The model under review builds one solid part; all positions refer to its coordinate system, in mm. Coordinates: 2 decimals unless noted, no trailing zeros. Answer in a Markdown table with one row per item.
```python
from build123d import *

# Parameters (mm, degrees)
SKETCH1_W           = 359.156
SKETCH1_H           = 127
BOSS_EXTRUDE1_DEPTH = 19.05
CUT_EXTRUDE1_REACH  = 21.05
SKETCH2_R           = 2.85115
CUT_EXTRUDE2_REACH  = 21.05
SKETCH3_R           = 3.175


with BuildPart() as part:
    # Sketch1 → Boss-Extrude1 (new body)
    with BuildSketch(Plane.XY):
        with Locations((179.578, 63.5)):
            Rectangle(SKETCH1_W, SKETCH1_H)
    extrude(amount=BOSS_EXTRUDE1_DEPTH)

    # Sketch2 → Cut-Extrude1 (cut, up to next)
    with BuildSketch(Plane.XY.offset(19.05), mode=Mode.PRIVATE) as cut_extrude1_sk1:
        with Locations((48.82515, 82.96275)):
            Circle(SKETCH2_R)
    cut_extrude1_tool1 = extrude(cut_extrude1_sk1.sketch, amount=-CUT_EXTRUDE1_REACH, mode=Mode.PRIVATE) & part.part
    add(cut_extrude1_tool1.solids().sort_by_distance((48.82515, 82.96275, 19.05))[0], mode=Mode.SUBTRACT)
    # Sketch2 → Cut-Extrude1 (cut, up to next)
    with BuildSketch(Plane.XY.offset(19.05), mode=Mode.PRIVATE) as cut_extrude1_sk2:
        with Locations((48.82515, 107.53725)):
            Circle(SKETCH2_R)
    cut_extrude1_tool2 = extrude(cut_extrude1_sk2.sketch, amount=-CUT_EXTRUDE1_REACH, mode=Mode.PRIVATE) & part.part
    add(cut_extrude1_tool2.solids().sort_by_distance((48.82515, 107.53725, 19.05))[0], mode=Mode.SUBTRACT)
    # Sketch2 → Cut-Extrude1 (cut, up to next)
    with BuildSketch(Plane.XY.offset(19.05), mode=Mode.PRIVATE) as cut_extrude1_sk3:
        with Locations((81.47685, 107.53725)):
            Circle(SKETCH2_R)
    cut_extrude1_tool3 = extrude(cut_extrude1_sk3.sketch, amount=-CUT_EXTRUDE1_REACH, mode=Mode.PRIVATE) & part.part
    add(cut_extrude1_tool3.solids().sort_by_distance((81.47685, 107.53725, 19.05))[0], mode=Mode.SUBTRACT)
    # Sketch2 → Cut-Extrude1 (cut, up to next)
    with BuildSketch(Plane.XY.offset(19.05), mode=Mode.PRIVATE) as cut_extrude1_sk4:
        with Locations((81.47685, 82.96275)):
            Circle(SKETCH2_R)
    cut_extrude1_tool4 = extrude(cut_extrude1_sk4.sketch, amount=-CUT_EXTRUDE1_REACH, mode=Mode.PRIVATE) & part.part
    add(cut_extrude1_tool4.solids().sort_by_distance((81.47685, 82.96275, 19.05))[0], mode=Mode.SUBTRACT)

    # Sketch3 → Cut-Extrude2 (cut, up to next)
    with BuildSketch(Plane(origin=(0, 0, 0), x_dir=(-1, 0, 0), z_dir=(0, 0, -1)), mode=Mode.PRIVATE) as cut_extrude2_sk1:
        with Locations((-65.151, 117.475)):
            Circle(SKETCH3_R)
    cut_extrude2_tool1 = extrude(cut_extrude2_sk1.sketch, amount=-CUT_EXTRUDE2_REACH, mode=Mode.PRIVATE) & part.part
    add(cut_extrude2_tool1.solids().sort_by_distance((65.151, 117.475, 0))[0], mode=Mode.SUBTRACT)


solid = part.part
```
Item 1: Mouldability with a two-part tool opening along X and no side actions: class faces 1 (the face through (359.156, 63, 9)), 2 (the face through (65.839, 114.376, 9.392)), 3 (the face through (177, 0, 9)) as +X half, -X half, draft (parallel to the pull), parting line (faces both ways), or undercut.
Check values:
| item | result |
|---|---|
| face 1 | +X half |
| face 2 | undercut |
| face 3 | draft |
Item 2: To check wall thickness, follow line 1 (X direction, y = 108, z = 12.5). State the ranges of the line that lie inside material, in increasing order. Write a range as from..to.
Check values:
| item | result |
|---|---|
| line 1 | 0..46.01, 51.64..78.66, 84.29..359.16 |
Item 3: Clearance check with a flat-ended pin moving along its axis: pin 1 Ø4.5 at (x, y) = (81.48, 82.96) entering from -Z. State where the tip first meets the part, or that it passes through.
Check values:
| item | result |
|---|---|
| pin 1 | through |
